from build123d import *

# Parameters (mm, degrees)
SKETCH_1_R      = 4
SKETCH_1_R_2    = 1.5
EXTRUDE_1_DEPTH = 3


with BuildPart() as part:
    # 草图1 → 凸台-拉伸1 (new body)
    with BuildSketch(Plane.XY):
        with BuildLine():
            Line((-12, -3.5), (-8.5, -3.5))
            ThreePointArc((-8.5, -3.5), (-4.964466094, -4.964466094), (-3.5, -8.5))
            Line((-3.5, -8.5), (-3.5, -35))
            ThreePointArc((-3.5, -35), (0, -38.5), (3.5, -35))
            Line((3.5, -35), (3.5, -8.5))
            ThreePointArc((3.5, -8.5), (4.964466094, -4.964466094), (8.5, -3.5))
            Line((8.5, -3.5), (12, -3.5))
            ThreePointArc((12, -3.5), (15.5, 0), (12, 3.5))
            Line((12, 3.5), (8.470537173, 3.5))
            ThreePointArc((8.470537173, 3.5), (6.561130633, 3.878943122), (4.941146684, 4.958333333))
            ThreePointArc((4.941146684, 4.958333333), (0, 7), (-4.941146684, 4.958333333))
            ThreePointArc((-4.941146684, 4.958333333), (-6.561130633, 3.878943122), (-8.470537173, 3.5))
            Line((-8.470537173, 3.5), (-12, 3.5))
            ThreePointArc((-12, 3.5), (-15.5, 0), (-12, -3.5))
        make_face()
        Circle(SKETCH_1_R, mode=Mode.SUBTRACT)
        with Locations((-12, 0)):
            Circle(SKETCH_1_R_2, mode=Mode.SUBTRACT)
        with Locations((0, -35)):
            Circle(SKETCH_1_R_2, mode=Mode.SUBTRACT)
        with Locations((12, 0)):
            Circle(SKETCH_1_R_2, mode=Mode.SUBTRACT)
    extrude(amount=EXTRUDE_1_DEPTH)


solid = part.part
The listing builds one solid part. Answer for the finished solid, in the listing's coordinates (mm). A direction names the side the tool comes from. Round coordinates to 2 decimals unless told otherwise and drop trailing zeros. Order: outer loops, then holes, each group sorted by start corner. A loop starts at its lowest first (then second) coordinate and runs counter-clockwise, first axis right, second up. Notation, with made-up numbers: (32.5, -20.5) -> (49.5, -20.5) arc R16 cw to (49.5, -15.5) -> close; hole circle Ø4 at (-9.75, 2.25). An arc over 180 degrees is marked (long way). One line per item, written item: value.
Item 1: For a pull along X with two mould halves and no side action, classify faces 1 (the cylindrical face through (-15.5, 0.1, 1.5)), 2 (the flat face through (10, -3.5, 1)), 3 (the cylindrical face through (10.5, 0.07, 1.48)) as released by +X, released by -X, zero draft, split by the parting line, or undercut.
Taken from the geometry:
face 1: released by -X
face 2: zero draft
face 3: undercut
Item 2: Find section C-C, the plane z = 1.7. Give the vertices of the cut face in (x, y).
Taken from the geometry:
outline: (-12, -3.5) -> (-8.5, -3.5) arc R5 cw to (-3.5, -8.5) -> (-3.5, -35) arc R3.5 ccw to (3.5, -35) -> (3.5, -8.5) arc R5 cw to (8.5, -3.5) -> (12, -3.5) arc R3.5 ccw to (12, 3.5) -> (8.47, 3.5) arc R5 cw to (4.94, 4.96) arc R7 ccw to (-4.94, 4.96) arc R5 cw to (-8.47, 3.5) -> (-12, 3.5) arc R3.5 ccw to start; hole circle Ø3 at (-12, 0); hole circle Ø8 at (0, 0); hole circle Ø3 at (0, -35); hole circle Ø3 at (12, 0)
Item 3: Find section A-A, the plane x = 0. Give the vertices of the cut face in (y, z).
Taken from the geometry:
outline: (-38.5, 0) -> (-36.5, 0) -> (-36.5, 3) -> (-38.5, 3) -> close; (-33.5, 0) -> (-4, 0) -> (-4, 3) -> (-33.5, 3) -> close; (4, 0) -> (7, 0) -> (7, 3) -> (4, 3) -> close
Item 4: Find section D-D, the plane x = 12.5. Give the vertices of the cut face in (y, z).
Taken from the geometry:
outline: (-3.46, 0) -> (-1.41, 0) -> (-1.41, 3) -> (-3.46, 3) -> close; (1.41, 0) -> (3.46, 0) -> (3.46, 3) -> (1.41, 3) -> close
Item 5: Find section B-B, the plane y = 0. Give the vertices of the cut face in (x, z).
Taken from the geometry:
outline: (-15.5, 0) -> (-13.5, 0) -> (-13.5, 3) -> (-15.5, 3) -> close; (-10.5, 0) -> (-4, 0) -> (-4, 3) -> (-10.5, 3) -> close; (4, 0) -> (10.5, 0) -> (10.5, 3) -> (4, 3) -> close; (13.5, 0) -> (15.5, 0) -> (15.5, 3) -> (13.5, 3) -> close
Item 6: Given P1, Ø1.5, axis at x = -7, z = 0.5, coming from the -Y side; P2, Ø0.9, axis at x = 10, z = 1.5, coming from the -Y side; P3, Ø0.9, axis at y = -21.5, z = 1, coming from the +X side; P4, Ø6.5, axis at x = 0, y = 0, coming from the +Z side, each flat-ended and moving along its own axis, determine where each tip first touches the part or whether it passes through.
Taken from the geometry:
P1: stops at y = -4.03
P2: stops at y = -3.5
P3: stops at x = 3.5
P4: passes through
Item 7: For faces 4 (the flat face through (-3.5, -22, 1)), 5 (the flat face through (3.5, -22, 1)), 6 (the cylindrical face through (0, 7, 1)), 7 (the flat face through (10, 3.5, 1)), 8 (the flat face through (-10, 3.5, 1)), determine the directions among +Z, -Z, +X, -X, +Y, -Y from which every point of the face is accessible in a straight line to the end or side of a thin tool.
Taken from the geometry:
face 4: +Z, -Z, -X, -Y
face 5: +Z, -Z, +X, -Y
face 6: +Z, -Z, +Y
face 7: +Z, -Z, +X, +Y
face 8: +Z, -Z, -X, +Y
Item 8: Straight lines are drawn through the part: L1, parallel to Y at x = 0, z = 2.3; L2, parallel to Y at x = 12, z = 2.15; L3, parallel to X at y = 0.5, z = 1.9. For each, find the intervals that lie inside material, in ascending order.
Taken from the geometry:
L1: y = -38.5 to -36.5, -33.5 to -4, 4 to 7
L2: y = -3.5 to -1.5, 1.5 to 3.5
L3: x = -15.46 to -13.41, -10.59 to -3.97, 3.97 to 10.59, 13.41 to 15.46
